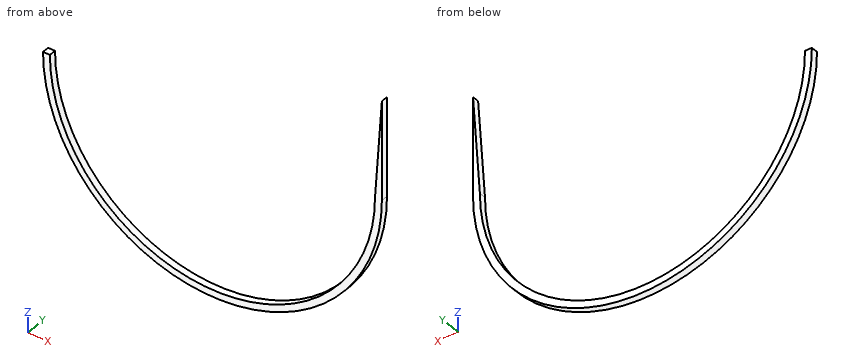
from build123d import *

# Parameters (mm, degrees)
BOSS_EXTRUDE1_DEPTH = 5.7


with BuildPart() as part:
    # Sketch1 → Boss-Extrude1 (new body)
    with BuildSketch(Plane(origin=(0, 0, 0), x_dir=(1, 0, 0), z_dir=(0, 1, 0))):
        with BuildLine():
            Line((-280.7, 115), (-275, 115))
            ThreePointArc((-275, 115), (-140.35, 249.65), (-5.7, 115))
            Line((-5.7, 115), (0, 33.358770855))
            Line((0, 33.358770855), (0, 115))
            ThreePointArc((0, 115), (-140.35, 255.35), (-280.7, 115))
        make_face()
    extrude(amount=BOSS_EXTRUDE1_DEPTH)


solid = part.part
Geometry check sheet. Reference: the model listing, model coordinates, mm. Round coordinates to 2 decimals unless told otherwise and drop trailing zeros. Write each loop counter-clockwise with the first axis right and the second up, starting at its lowest first coordinate (ties: lowest second). Pieces come first, ordered by that corner, then holes.
Item 1: Go/stop test with flat-tipped pins: pin 1 Ø2 at (x, y) = (-112, 1.5) entering from +Z; pin 2 Ø2 at (x, y) = (-71, 5) entering from -Z; pin 3 Ø2 at (x, y) = (-144.5, 4) entering from -Z. Record where each tip stops, or that it passes through.
Determined:
pin 1: stops at z = -246.41
pin 2: stops at z = -237.58
pin 3: stops at z = -255.31
Item 2: Section check A-A (z = -171.5). Record the boundary of the cut face in (x, y).
Determined:
outline: (-268.83, 0) - (-262.57, 0) - (-262.57, 5.7) - (-268.83, 5.7) - close; (-18.13, 0) - (-11.87, 0) - (-11.87, 5.7) - (-18.13, 5.7) - close
Item 3: Section check B-B (y = 4.65). Record the boundary of the cut face in (x, z).
Determined:
outline: (-280.7, -115) arc R140.35 ccw to (0, -115) - (0, -33.36) - (-5.7, -115) arc R134.65 cw to (-275, -115) - close
Item 4: Section check D-D (z = -104). Record the boundary of the cut face in (x, y).
Determined:
outline: (-4.93, 0) - (0, 0) - (0, 5.7) - (-4.93, 5.7) - close
Item 5: Material ranges on line 1 along X through (y, z) = (1, -215); line 2 along X through (y, z) = (1.95, -129); line 3 along Z through (x, y) = (-206.5, 2.15), recorded low to high.
Determined:
line 1: x = -238.83 to -230.52, -50.18 to -41.87
line 2: x = -280 to -274.27, -6.43 to -0.7
line 3: z = -238.78 to -232.28
Item 6: Section check C-C (x = -140.35). Record the boundary of the cut face in (y, z), plus the area to 3 significant figures.
Determined:
outline: (0, -255.35) - (5.7, -255.35) - (5.7, -249.65) - (0, -249.65) - close
area: 32.5 mm2
